Could you check a few things on this drawing? It's one solid part, dimensions in mm from its lowest x, y, z. Coordinates: 2 decimals unless noted, no trailing zeros. Write each loop counter-clockwise with the first axis right and the second up, starting at its lowest first coordinate (ties: lowest second). Pieces come first, ordered by that corner, then holes.
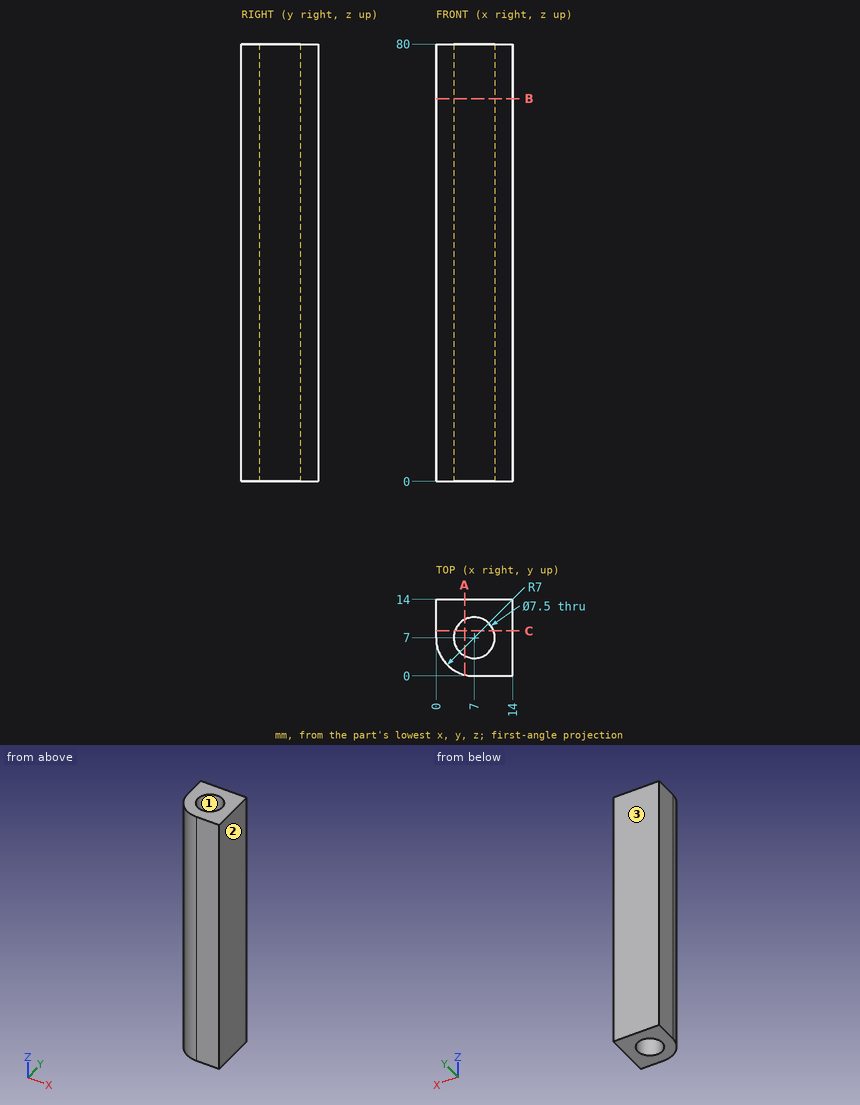
1) We'd pull the mould along X, two halves only. Please class the marked faces 1, 2 and 3: pulls with the +X half, pulls with the -X half, needs draft (parallel to the pull), parting line crosses it, or undercut.
Values follow:
face 1: undercut
face 2: pulls with the +X half
face 3: needs draft
2) Imagine slicing it at A-A on x = 5.25. Please give me the cut outline in (y, z).
Values follow:
outline: (0.22, 0) - (3.68, 0) - (3.68, 80) - (0.22, 80) - close; (10.32, 0) - (14, 0) - (14, 80) - (10.32, 80) - close
3) Will these pins go through, and if not, where does the flat tip stop? pin 1 (4.5 mm diameter, centred on x = 7, y = 7, fed in from +Z); pin 2 (1 mm diameter, centred on x = 2, y = 1.5, fed in from +Z).
Values follow:
pin 1: passes through
pin 2: stops at z = 80
4) I need wall thicknesses on probe 1 along Y at (x, z) = (7, 36); probe 2 along Y at (x, z) = (4.5, 27); probe 3 along X at (y, z) = (4.25, 24). Which ranges of each line are inside material? Lowest first, please.
Values follow:
probe 1: y = 0 to 3.25, 10.75 to 14
probe 2: y = 0.46 to 4.2, 9.8 to 14
probe 3: x = 0.56 to 4.45, 9.55 to 14
5) Imagine slicing it at B-B on z = 70. Please give me the cut outline in (x, y).
Values follow:
outline: (0, 7) arc R7 ccw to (7, 0) - (14, 0) - (14, 14) - (0, 14) - close; hole circle Ø7.5 at (7, 7)
6) Imagine slicing it at C-C on y = 8.25. Please give me the cut outline in (x, z).
Values follow:
outline: (0, 0) - (3.46, 0) - (3.46, 80) - (0, 80) - close; (10.54, 0) - (14, 0) - (14, 80) - (10.54, 80) - close
